Verification items for the finished model (mm, model axes). A direction names the side the tool comes from. Round coordinates to 2 decimals unless told otherwise and drop trailing zeros. Write each loop counter-clockwise with the first axis right and the second up, starting at its lowest first coordinate (ties: lowest second). Pieces come first, ordered by that corner, then holes. Notation, with made-up numbers: M 6,12 L 48,12 A25 cw 48,41 Z; hole C 19,-25.5 d1. An arc over 180 degrees is marked long. One line per question, with ' | ' between items.
from build123d import *

# Parameters (mm, degrees)
CUT_EXTRUDE3_DEPTH      = 10
CUT_EXTRUDE3_DEPTH_BACK = 10
CUT_EXTRUDE4_DEPTH      = 10
CUT_EXTRUDE4_DEPTH_BACK = 10
SKETCH7_R               = 4
FILLET1_R               = 0.15
SKETCH8_R               = 1
CUT_EXTRUDE5_DEPTH      = 5
CHAMFER1_SIZE           = 0.05


with BuildPart() as part:
    # Sketch5 → Revolve2 (revolve)
    with BuildSketch(Plane(origin=(0, 0, 0), x_dir=(1, 0, 0), z_dir=(0, 1, 0)), mode=Mode.PRIVATE) as revolve2_sk:
        with BuildLine():
            Line((-1.5, -15), (0, -15))
            Line((0, -15), (0, 5))
            ThreePointArc((0, 5), (-4.657160695, 1.819575298), (-3.389621823, -3.675658294))
            ThreePointArc((-3.389621823, -3.675658294), (-2.089993468, -5.412512495), (-1.5, -7.5))
            Line((-1.5, -7.5), (-1.5, -15))
        make_face()
    revolve(revolve2_sk.sketch.rotate(Axis((0, 0, 15), (0, 0, -1)), 180), axis=Axis((0, 0, 15), (0, 0, -1)))

    # Sketch6 → Cut-Extrude3 (cut, two sides: drawn at the far end of the back side and taken through both)
    with BuildSketch(Plane(origin=(0, 0, 0), x_dir=(0, 0, -1), z_dir=(1, 0, 0)).offset(-CUT_EXTRUDE3_DEPTH_BACK)):
        with BuildLine():
            Line((-19.567307599, 10.758838429), (14.902121045, 10.758838429))
            Line((14.902121045, 10.758838429), (14.902121045, 1.875))
            Line((14.902121045, 1.875), (-5.303377511, 1.875))
            ThreePointArc((-5.303377511, 1.875), (-6.806906508, 2.106415246), (-8.171259692, 2.779239779))
            Line((-8.171259692, 2.779239779), (-19.567307599, 10.758838429))
        make_face()
        with BuildLine():
            Line((-8.171259692, -2.779239779), (-19.567307599, -10.758838429))
            Line((-19.567307599, -10.758838429), (14.902121045, -10.758838429))
            Line((14.902121045, -10.758838429), (14.902121045, -1.875))
            Line((14.902121045, -1.875), (-5.303377511, -1.875))
            ThreePointArc((-5.303377511, -1.875), (-6.806906508, -2.106415246), (-8.171259692, -2.779239779))
        make_face()
    extrude(amount=CUT_EXTRUDE3_DEPTH + CUT_EXTRUDE3_DEPTH_BACK, mode=Mode.SUBTRACT)

    # Sketch7 → Cut-Extrude4 (cut, two sides: drawn at the far end of the back side and taken through both)
    with BuildSketch(Plane(origin=(0, 0, 0), x_dir=(1, 0, 0), z_dir=(0, 1, 0)).offset(-CUT_EXTRUDE4_DEPTH_BACK)):
        with Locations(Location((0, 0, 0), (0, 0, 90))):
            Circle(SKETCH7_R)
    extrude(amount=CUT_EXTRUDE4_DEPTH + CUT_EXTRUDE4_DEPTH_BACK, mode=Mode.SUBTRACT)

    # Fillet1
    fillet1_edges = [part.edges().sort_by_distance(p)[0] for p in [
        (1.909227576, 1.875, 4.46296456),
        (-1e-09, 1.902919108, 5.831024745),
        (-1.909227576, 1.875, 4.46296456),
        (0, 1.875, -4.635124054),
        (0, 1.875, 4),
    ]]
    fillet(fillet1_edges, radius=FILLET1_R)

    # Sketch8 → Cut-Extrude5 (cut)
    with BuildSketch(Plane.XY.offset(15)):
        Circle(SKETCH8_R)
    extrude(amount=-CUT_EXTRUDE5_DEPTH, mode=Mode.SUBTRACT)

    # Chamfer1
    chamfer1_edges = [part.edges().sort_by_distance(p)[0] for p in [
        (-1.5, 0, 15),
        (-1, 0, 15),
    ]]
    chamfer(chamfer1_edges, length=CHAMFER1_SIZE)


solid = part.part
1. Thickness scan on line 1 (X direction, y = 0.1, z = 13.5); line 2 (X direction, y = -0.4, z = 11); line 3 (Y direction, x = -1.5, z = 4) (3 decimals). Record the ranges inside material, lowest first.
Results:
line 1: x = -1.5 to -0.99, 0.99 to 1.5 | line 2: x = -1.45 to -0.92, 0.92 to 1.45 | line 3: y = -1.875 to 1.875
2. Section check A-A, the plane y = 0. Record the cut outline in (x, z).
Results:
outline: M -3.39,3.68 A5 ccw long 3.39,3.68 A5.95 cw 1.5,7.5 L 1.5,14.95 L 1.45,15 L 1.05,15 L 1,14.95 L 1,10 L -1,10 L -1,14.95 L -1.05,15 L -1.45,15 L -1.5,14.95 L -1.5,7.5 A5.95 cw Z; hole C 0,0 d8
3. Mould release check, pull along Y, two halves, no side actions. Record for faces 3 (the face through (0, -1, 13)), 4 (the face through (1.43, -0.45, 11.28)), 5 (the face through (-2, 1.875, 4)), 6 (the face through (0, 0, 10)): pulls with the +Y half, pulls with the -Y half, needs draft (parallel to the pull), parting line crosses it, or undercut.
Results:
face 3: undercut | face 4: parting line crosses it | face 5: pulls with the +Y half | face 6: undercut
4. Go/stop test with a flat-tipped pin: P1, Ø1.5, axis at x = 3, y = -1.5, coming from the +Z side. Record where the tip stops, or that it passes through.
Results:
P1: stops at z = 4.56
5. Section check B-B, the plane z = 8.5. Record the cut outline in (x, y), then the cut area to 3 significant figures.
Results:
outline: C 0,0 d3 | area: 7.07 mm2
6. Tool access check on faces 1 (the face through (3.905, -0.1, 0.867)), 2 (the face through (-2, -1.875, 4)). Record the directions out of +Z, -Z, +X, -X, +Y, -Y that give a thin tool (end or side, any length) a straight path to the whole face; none if there is none.
Results:
face 1: +Y, -Y | face 2: -Z, +X, -X, -Y
